from build123d import *

# Parameters (mm, degrees)
SKETCH_1_W          = 85
SKETCH_1_H          = 30
EXTRUDE_1_DEPTH     = 45
SKETCH_2_W          = 85
SKETCH_2_H          = 26
CUT_EXTRUDE_1_DEPTH = 28
SKETCH_3_W          = 85
SKETCH_3_H          = 13
CUT_EXTRUDE_3_DEPTH = 13
SKETCH_4_W          = 10
SKETCH_4_H          = 2
CUT_EXTRUDE_4_DEPTH = 31
FILLET_1_R          = 3
SKETCH_5_R          = 1.6
CUT_EXTRUDE_5_DEPTH = 8
SKETCH_6_W          = 5.7
SKETCH_6_H          = 2.3
CUT_EXTRUDE_6_DEPTH = 31


with BuildPart() as part:
    # 草图1 → 凸台-拉伸1 (new body)
    with BuildSketch(Plane(origin=(0, 0, 0), x_dir=(1, 0, 0), z_dir=(0, 1, 0))):
        Rectangle(SKETCH_1_W, SKETCH_1_H)
    extrude(amount=EXTRUDE_1_DEPTH)

    # 草图2 → 切除-拉伸1 (cut)
    with BuildSketch(Plane(origin=(0, 45, 0), x_dir=(1, 0, 0), z_dir=(0, 1, 0))):
        Rectangle(SKETCH_2_W, SKETCH_2_H)
    extrude(amount=-CUT_EXTRUDE_1_DEPTH, mode=Mode.SUBTRACT)

    # 草图3 → 切除-拉伸3 (cut)
    with BuildSketch(Plane(origin=(0, 17, 0), x_dir=(1, 0, 0), z_dir=(0, 1, 0))):
        with Locations((0, -2.5)):
            Rectangle(SKETCH_3_W, SKETCH_3_H)
    extrude(amount=-CUT_EXTRUDE_3_DEPTH, mode=Mode.SUBTRACT)

    # 草图4 → 切除-拉伸4 (cut, through all)
    with BuildSketch(Plane.XY.offset(15)):
        with Locations((-17.315675278, 14)):
            Rectangle(SKETCH_4_W, SKETCH_4_H)
        with Locations((17.315675278, 14)):
            Rectangle(SKETCH_4_W, SKETCH_4_H)
    extrude(amount=-CUT_EXTRUDE_4_DEPTH, mode=Mode.SUBTRACT)

    # 圆角1
    fillet_1_edges = [part.edges().sort_by_distance(p)[0] for p in [
        (0, 17, 13),
        (0, 17, -13),
        (0, 4, -4),
        (0, 4, 9),
    ]]
    fillet(fillet_1_edges, radius=FILLET_1_R)

    # 草图5 → 切除-拉伸5 (cut)
    with BuildSketch(Plane.XZ):
        with Locations((-30, 11.5)):
            Circle(SKETCH_5_R)
        with Locations((-30, -11.5)):
            Circle(SKETCH_5_R)
        with Locations((30, -11.5)):
            Circle(SKETCH_5_R)
        with Locations((30, 11.5)):
            Circle(SKETCH_5_R)
    extrude(amount=-CUT_EXTRUDE_5_DEPTH, mode=Mode.SUBTRACT)

    # 草图6 → 切除-拉伸6 (cut, through all)
    with BuildSketch(Plane.XY.offset(15)):
        with Locations((-30, 5.15)):
            Rectangle(SKETCH_6_W, SKETCH_6_H)
        with Locations((30, 5.15)):
            Rectangle(SKETCH_6_W, SKETCH_6_H)
    extrude(amount=-CUT_EXTRUDE_6_DEPTH, mode=Mode.SUBTRACT)


solid = part.part
Can you work these out from the model? Positions are in its coordinate system, mm. A direction names the side the tool comes from. Round coordinates to 2 decimals unless told otherwise and drop trailing zeros. Write each loop counter-clockwise with the first axis right and the second up, starting at its lowest first coordinate (ties: lowest second). Pieces come first, ordered by that corner, then holes. Notation, with made-up numbers: M 75.5,-14.5 L 113.5,-14.5 A31 cw 113.5,14.5 Z; hole C 35.5,8 d9. An arc over 180 degrees is marked long. Use CSV: the item, a comma, the result in double quotes.
(1) We'd pull the mould along Z, two halves only. Please class faces 1 (the flat face through (17, 15, 12)), 2 (the flat face through (-1, 22, 15)), 3 (the cylindrical face through (0.59, 4.9, -3.14)): +Z half, -Z half, draft (parallel to the pull), parting line (faces both ways), or undercut.
Check values:
face 1,"draft"
face 2,"+Z half"
face 3,"undercut"
(2) Imagine slicing it at C-C (y = 34). Write out the boundary of the cut face in (x, z), plus the area to 3 significant figures.
Check values:
outline,"M -42.5,-15 L 42.5,-15 L 42.5,-13 L -42.5,-13 Z; M -42.5,13 L 42.5,13 L 42.5,15 L -42.5,15 Z"
area,"340 mm^2"
(3) I need wall thicknesses on line 1 along Z through (x, y) = (30, 7.5); line 2 along Z through (x, y) = (27.5, 8.5); line 3 along Z through (x, y) = (-30, 1.6). Which ranges of each line are inside material? Lowest first, please.
Check values:
line 1,"-15 to -13.1, -9.9 to -4, 9 to 9.9, 13.1 to 15"
line 2,"-15 to -4, 9 to 15"
line 3,"-15 to -13.1, -9.9 to 9.9, 13.1 to 15"
(4) Imagine slicing it at B-B (z = -8.5). Write out the boundary of the cut face in (x, y), plus the area to 3 significant figures.
Check values:
outline,"M -42.5,0 L 42.5,0 L 42.5,17 L -42.5,17 Z; hole M -32.85,4 L -27.15,4 L -27.15,6.3 L -32.85,6.3 Z; hole M -22.32,13 L -12.32,13 L -12.32,15 L -22.32,15 Z; hole M 12.32,13 L 22.32,13 L 22.32,15 L 12.32,15 Z; hole M 27.15,4 L 32.85,4 L 32.85,6.3 L 27.15,6.3 Z"
area,"1,380 mm^2"
(5) Imagine slicing it at A-A (y = 14). Write out the boundary of the cut face in (x, z).
Check values:
outline,"M -42.5,-15 L -22.32,-15 L -22.32,-4 L -42.5,-4 Z; M -42.5,9 L -22.32,9 L -22.32,15 L -42.5,15 Z; M -12.32,-15 L 12.32,-15 L 12.32,-4 L -12.32,-4 Z; M -12.32,9 L 12.32,9 L 12.32,15 L -12.32,15 Z; M 22.32,-15 L 42.5,-15 L 42.5,-4 L 22.32,-4 Z; M 22.32,9 L 42.5,9 L 42.5,15 L 22.32,15 Z"
(6) On a 3-axis mill with a long thin cutter (end or side, diameter ignored), from which of +Z, -Z, +X, -X, +Y, -Y can I reach the whole of each face in a straight line? I mean faces 4 (the flat face through (-32.85, 5, -9)), 5 (the flat face through (-1, 22, -15)), 6 (the flat face through (-1, 4, 0)), 7 (the cylindrical face through (-31.27, 1.97, -12.47)), 8 (the cylindrical face through (0.59, 17.86, 12.1)). Say none if no direction works.
Check values:
face 4,"+Z, -Z"
face 5,"-Z, +X, -X, +Y, -Y"
face 6,"none"
face 7,"-Y"
face 8,"+X, -X, +Y"
(7) Imagine slicing it at D-D (x = -9). Write out the boundary of the cut face in (y, z), plus the area to 3 significant figures.
Check values:
outline,"M 0,-15 L 45,-15 L 45,-13 L 20,-13 A3 cw 17,-10 L 17,-4 L 7,-4 A3 cw 4,-1 L 4,6 A3 cw 7,9 L 17,9 L 17,10 A3 cw 20,13 L 45,13 L 45,15 L 0,15 Z"
area,"461 mm^2"
(8) I'm going to push flat-ended pins straight in: pin 1 (12 mm diameter, centred on x = -2, z = -6, fed in from +Y); pin 2 (3 mm diameter, centred on x = 18, z = -8, fed in from +Y); pin 3 (6 mm diameter, centred on y = 21, z = 0, fed in from -X); pin 4 (1 mm diameter, centred on x = 21, z = -1.5, fed in from +Y). Where does each tip first touch, or does it pass through?
Check values:
pin 1,"y = 17.76"
pin 2,"y = 17"
pin 3,"through"
pin 4,"y = 4.17"
